from build123d import *

# Parameters (mm, degrees)
F2_R      = 4.7625
F3_DEPTH  = 14.605
F4_R      = 1.6002
F5_DEPTH  = 10.16
F6_R      = 4.7752
F7_DEPTH  = 14.605
F8_R      = 3.728231
F9_DEPTH  = 14.605
F10_R     = 1.6002
F11_DEPTH = 10.16
F12_SIZE  = 2.159
F13_R     = 1.778


with BuildPart() as f1:
    # F0 (on Right) → F1 (revolve)
    with BuildSketch(Plane.YZ):
        with BuildLine():
            Line((0, 30.265944), (0, 0))
            Line((0, 0), (2.686187, 0))
            ThreePointArc((2.686187, 0), (13.141494, 8.903682), (26.541598, 11.90805))
            Line((26.541598, 11.90805), (27.856382, 12.945489))
            Line((27.856382, 12.945489), (26.541598, 13.987607))
            ThreePointArc((26.541598, 13.987607), (15.736911, 15.929647), (6.995791, 22.570852))
            Line((6.995791, 22.570852), (6.995791, 30.265944))
            Line((6.995791, 30.265944), (0, 30.265944))
        make_face()
    revolve(axis=Axis((0, 0, 15.132972), (0, 0, -1)))

    # F2 (on face) → F3 (join)
    with BuildSketch(Plane.XY.offset(30.265944)):
        Circle(F2_R)
    extrude(amount=-F3_DEPTH)

    # F4 (on Top) → F5 (join)
    with BuildSketch(Plane.XY):
        Circle(F4_R)
    extrude(amount=F5_DEPTH)

    # F6 (on face) → F7 (join)
    with BuildSketch(Plane.XY.offset(30.265944)):
        Circle(F6_R)
    extrude(amount=-F7_DEPTH)

    # F8 (on face) → F9 (cut)
    with BuildSketch(Plane.XY.offset(30.265944)):
        Circle(F8_R)
    extrude(amount=-F9_DEPTH, mode=Mode.SUBTRACT)

    # F10 (on Top) → F11 (cut)
    with BuildSketch(Plane.XY):
        Circle(F10_R)
    extrude(amount=F11_DEPTH, mode=Mode.SUBTRACT)

    # F12
    f12_edges = [f1.edges().sort_by_distance(p)[0] for p in [
        (0, -6.995791, 30.265944),
    ]]
    chamfer(f12_edges, length=F12_SIZE)

    # F13
    f13_edges = [f1.edges().sort_by_distance(p)[0] for p in [
        (0, -2.686187, 0),
    ]]
    fillet(f13_edges, radius=F13_R)


solid = f1.part
Read the model definition and answer for the solid it produces. Units are mm, in the model's axes. A direction names the side the tool comes from. Coordinates: 2 decimals unless noted, no trailing zeros. Write item = value, one per line. Start each with the question number.
1) The mould has two halves that part along Y. Classify faces 3 (the face through (-4, 1, 30.266)), 4 (the face through (0, 0, 10.16)), 5 (the face through (0.22, -4.94, 30.16)), 6 (the face through (3.556, 1.12, 23.066)): pulls with the +Y half, pulls with the -Y half, needs draft (parallel to the pull), parting line crosses it, or undercut.
2) Given P1, Ø10, axis at x = 13.5, y = 6.5, coming from the -Z side; P2, Ø2, axis at x = 22, y = 16.5, coming from the -Z side; P3, Ø9.5, axis at x = 0, y = 0, coming from the -Z side; P4, Ø1, axis at x = -0.5, y = 0, coming from the -Z side, each flat-ended and moving along its own axis, determine where each tip first touches the part or whether it passes through.
3) Find the intervals of material crossed by L1, parallel to Y at x = 0, z = 18.5; L2, parallel to Z at x = 11.5, y = 23.5; L3, parallel to Y at x = 0, z = 7, in increasing order. Write a range as from..to.
4) For faces 1 (the face through (-1.27, -0.974, 5.009)), 2 (the face through (0, 0, 15.661)), determine the directions among +Z, -Z, +X, -X, +Y, -Y from which every point of the face is accessible in a straight line to the end or side of a thin tool.
Result:
q1.face_3 = needs draft
q1.face_4 = undercut
q1.face_5 = parting line crosses it
q1.face_6 = undercut
q2.P1 = 7.07
q2.P2 = 11.91
q2.P3 = 0
q2.P4 = 10.16
q3.L1 = -11.28..-3.73, 3.73..11.28
q3.L2 = 11.91..13.97
q3.L3 = -9.88..-1.6, 1.6..9.88
q4.face_1 = -Z
q4.face_2 = +Z
